Read the model definition and answer for the solid it produces. Units are mm, in the model's axes. Face numbers are marked on the shaded views. Give positions to 0.01 mm unless a question says otherwise; leave off trailing zeros. Write each loop counter-clockwise with the first axis right and the second up, starting at its lowest first coordinate (ties: lowest second). Pieces come first, ordered by that corner, then holes. Notation, with made-up numbers: M 39,-29 L 45,-29 A34 cw 45,10 Z; hole C 62,62.25 d5. An arc over 180 degrees is marked long. Put each result on its own line as item: value.
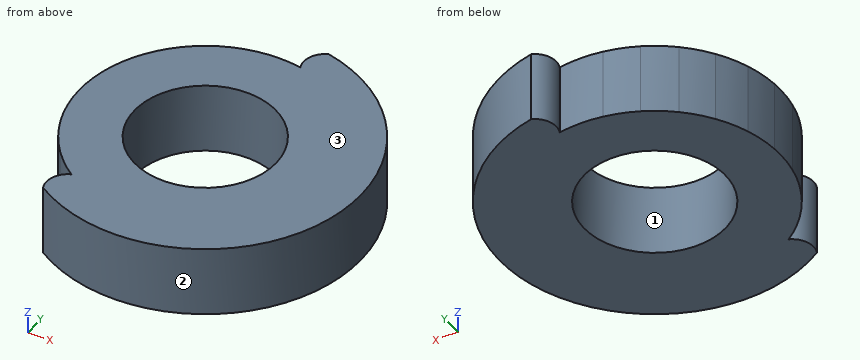
from build123d import *

# Parameters (mm, degrees)
SKETCH1_R           = 13.2
SKETCH1_R_2         = 6
BOSS_EXTRUDE1_DEPTH = 6
CUT_EXTRUDE1_DEPTH  = 7
SKETCH3_R           = 13.2
SKETCH3_R_2         = 6
BOSS_EXTRUDE2_DEPTH = 6
CUT_EXTRUDE2_DEPTH  = 7
CIRPATTERN2_COUNT   = 10
CIRPATTERN2_ANGLE   = 135


with BuildPart() as part:
    # Sketch1 → Boss-Extrude1 (new body)
    with BuildSketch(Plane.XY):
        Circle(SKETCH1_R)
        Circle(SKETCH1_R_2, mode=Mode.SUBTRACT)
    extrude(amount=BOSS_EXTRUDE1_DEPTH)

    # Sketch2 → Cut-Extrude1 (cut, through all)
    with BuildSketch(Plane.XY.offset(6)):
        with BuildLine():
            ThreePointArc((-2.819851171, 12.895287487), (0, 13.2), (2.819851171, 12.895287487))
            ThreePointArc((2.819851171, 12.895287487), (1.826256171, 11.910750525), (1.819851171, 10.512))
            ThreePointArc((1.819851171, 10.512), (0, 10.668364555), (-1.819851171, 10.512))
            ThreePointArc((-1.819851171, 10.512), (-1.826256171, 11.910750525), (-2.819851171, 12.895287487))
        make_face()
    extrude(amount=-CUT_EXTRUDE1_DEPTH, mode=Mode.SUBTRACT)

    # Sketch3 → Boss-Extrude2 (add)
    with BuildSketch(Plane.XY):
        Circle(SKETCH3_R)
        Circle(SKETCH3_R_2, mode=Mode.SUBTRACT)
    extrude(amount=BOSS_EXTRUDE2_DEPTH)

    # Sketch4 → Cut-Extrude2 (cut, through all)
    with BuildSketch(Plane.XY.offset(6)):
        with BuildLine():
            ThreePointArc((-2.819851171, 12.895287487), (0, 13.2), (2.819851171, 12.895287487))
            ThreePointArc((2.819851171, 12.895287487), (1.826256171, 11.910750525), (1.819851171, 10.512))
            ThreePointArc((1.819851171, 10.512), (0, 10.668364555), (-1.819851171, 10.512))
            ThreePointArc((-1.819851171, 10.512), (-1.826256171, 11.910750525), (-2.819851171, 12.895287487))
        make_face()
    cut_extrude2 = extrude(amount=-CUT_EXTRUDE2_DEPTH, mode=Mode.SUBTRACT)

    # CirPattern2: Cut-Extrude2 ×10 about axis
    cirpattern2_axis = Axis((0, 0, 0), (0, 0, 1))
    for i in range(1, CIRPATTERN2_COUNT):
        add(cut_extrude2.rotate(cirpattern2_axis, i * CIRPATTERN2_ANGLE / (CIRPATTERN2_COUNT - 1)), mode=Mode.SUBTRACT)


solid = part.part
(1) Section B-B on x = 0 is taken. Determine the outline of the cut face in (y, z), and give its area (3 significant figures).
Result:
outline: M -13.2,0 L -6,0 L -6,6 L -13.2,6 Z; M 6,0 L 10.67,0 L 10.67,6 L 6,6 Z
area: 71.2 mm²
(2) Section C-C on y = 0 is taken. Determine the outline of the cut face in (x, z).
Result:
outline: M -10.67,0 L -6,0 L -6,6 L -10.67,6 Z; M 6,0 L 13.2,0 L 13.2,6 L 6,6 Z
(3) Section A-A on z = 0.8 is taken. Determine the outline of the cut face in (x, y).
Result:
outline: M -7.12,-11.11 A13.2 ccw long 2.82,12.9 A1.83 ccw 1.82,10.51 A10.67 ccw -6.15,-8.72 A1.83 ccw Z; hole C 0,0 d12
(4) Given pin 1 Ø2 at (x, z) = (-6.5, 2) entering from -Y; pin 2 Ø2 at (x, y) = (3, -2.5) entering from +Z; pin 3 Ø3 at (x, z) = (2.5, 2.5) entering from +Y; pin 4 Ø1.5 at (y, z) = (4.5, 1) entering from -X, each flat-ended and moving along its own axis, determine where each tip first touches the part or whether it passes through.
Result:
pin 1: stops at y = -12
pin 2: passes through
pin 3: stops at y = 12.9
pin 4: stops at x = -9.99
(5) Straight lines are drawn through the part: line 1 along Y through (x, z) = (0, 3.45); line 2 along X through (y, z) = (-0.75, 3.3); line 3 along X through (y, z) = (5.5, 3). For each, find the intervals that lie inside material, in ascending order. Write a range as from..to.
Result:
line 1: y = -13.2..-6, 6..10.67
line 2: x = -10.64..-5.95, 5.95..13.18
line 3: x = -9.14..-2.4, 2.4..12
(6) For a pull along X with two mould halves and no side action, classify the marked faces 1, 2 and 3 as +X half, -X half, draft (parallel to the pull), parting line (faces both ways), or undercut.
Result:
face 1: undercut
face 2: parting line
face 3: draft
(7) Section D-D on x = 10.25 is taken. Determine the outline of the cut face in (y, z).
Result:
outline: M -8.32,0 L 8.32,0 L 8.32,6 L -8.32,6 Z
